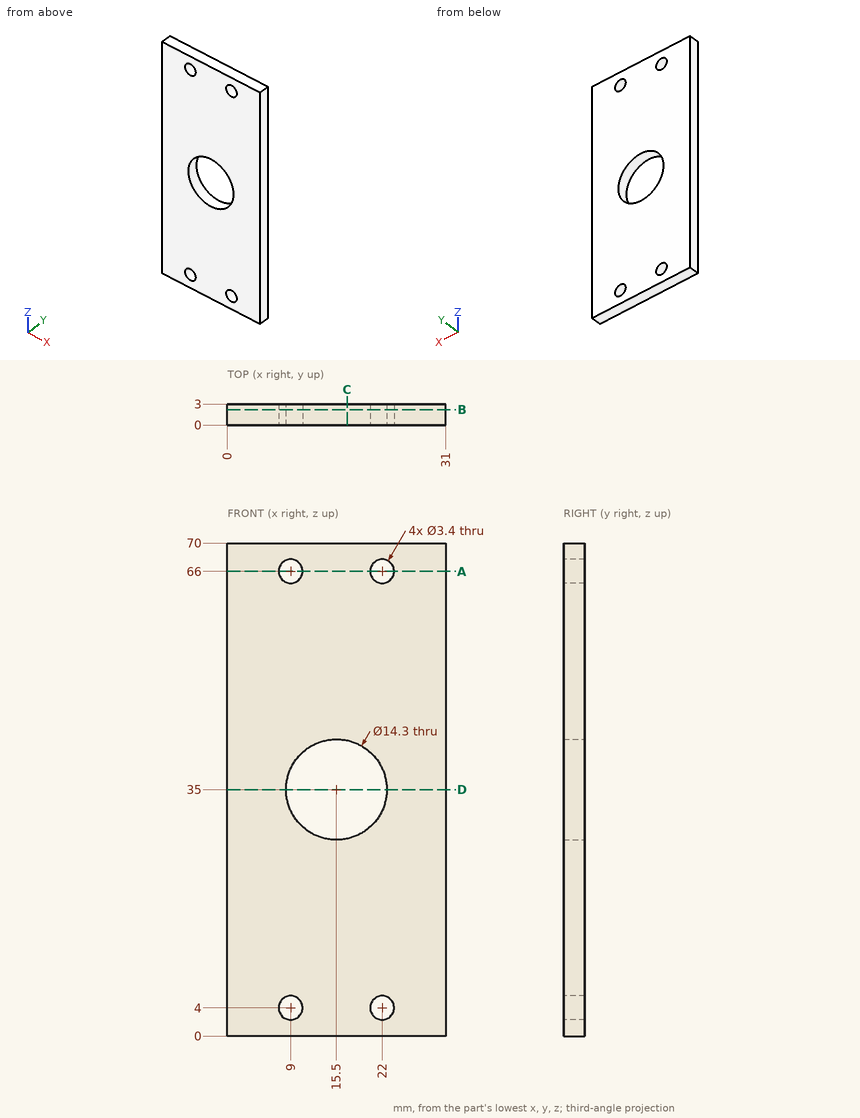
Print and shaded views of the part. All mm, measured from the part's lowest x, y and z. Round coordinates to 2 decimals unless told otherwise and drop trailing zeros. Write each loop counter-clockwise with the first axis right and the second up, starting at its lowest first coordinate (ties: lowest second). Pieces come first, ordered by that corner, then holes. Notation, with made-up numbers: (64, 55) -> (114, 55) arc R31 cw to (114, 84) -> close; hole circle Ø10 at (9, 3). An arc over 180 degrees is marked (long way). Answer in a Markdown table with one row per item. Add a question column.
Item 1: Drill centre lines: line 1 (X direction, y = 0.6, z = 4); line 2 (Z direction, x = 21, y = 2.5); line 3 (Z direction, x = 9, y = 2.15). Where is each one in solid material? Low to high. Write a range as from..to.
Item 2: Saw through at A-A, the plane z = 66. Write the cut outline in (x, y), then the cut area to 3 significant figures.
Item 3: Saw through at D-D, the plane z = 35. Write the cut outline in (x, y), then the cut area to 3 significant figures.
Item 4: Saw through at B-B, the plane y = 2.2. Write the cut outline in (x, z).
Item 5: Saw through at C-C, the plane x = 17. Write the cut outline in (y, z).
Item 6: Drop a flat-ended pin along its axis: pin 1 Ø11.5 at (x, z) = (15.5, 35) entering from +Y. Give the stop position or say it passes through.
Findings below:
| question | item | result |
|---|---|---|
| 1 | line 1 | x = 0..7.3, 10.7..20.3, 23.7..31 |
| 1 | line 2 | z = 0..2.63, 5.37..30.43, 39.57..64.63, 67.37..70 |
| 1 | line 3 | z = 0..2.3, 5.7..32.02, 37.98..64.3, 67.7..70 |
| 2 | outline | (0, 0) -> (7.3, 0) -> (7.3, 3) -> (0, 3) -> close; (10.7, 0) -> (20.3, 0) -> (20.3, 3) -> (10.7, 3) -> close; (23.7, 0) -> (31, 0) -> (31, 3) -> (23.7, 3) -> close |
| 2 | area | 72.6 mm^2 |
| 3 | outline | (0, 0) -> (8.35, 0) -> (8.35, 3) -> (0, 3) -> close; (22.65, 0) -> (31, 0) -> (31, 3) -> (22.65, 3) -> close |
| 3 | area | 50.1 mm^2 |
| 4 | outline | (0, 0) -> (31, 0) -> (31, 70) -> (0, 70) -> close; hole circle Ø3.4 at (9, 4); hole circle Ø3.4 at (9, 66); hole circle Ø14.3 at (15.5, 35); hole circle Ø3.4 at (22, 4); hole circle Ø3.4 at (22, 66) |
| 5 | outline | (0, 0) -> (3, 0) -> (3, 28.01) -> (0, 28.01) -> close; (0, 41.99) -> (3, 41.99) -> (3, 70) -> (0, 70) -> close |
| 6 | pin 1 | passes through |
